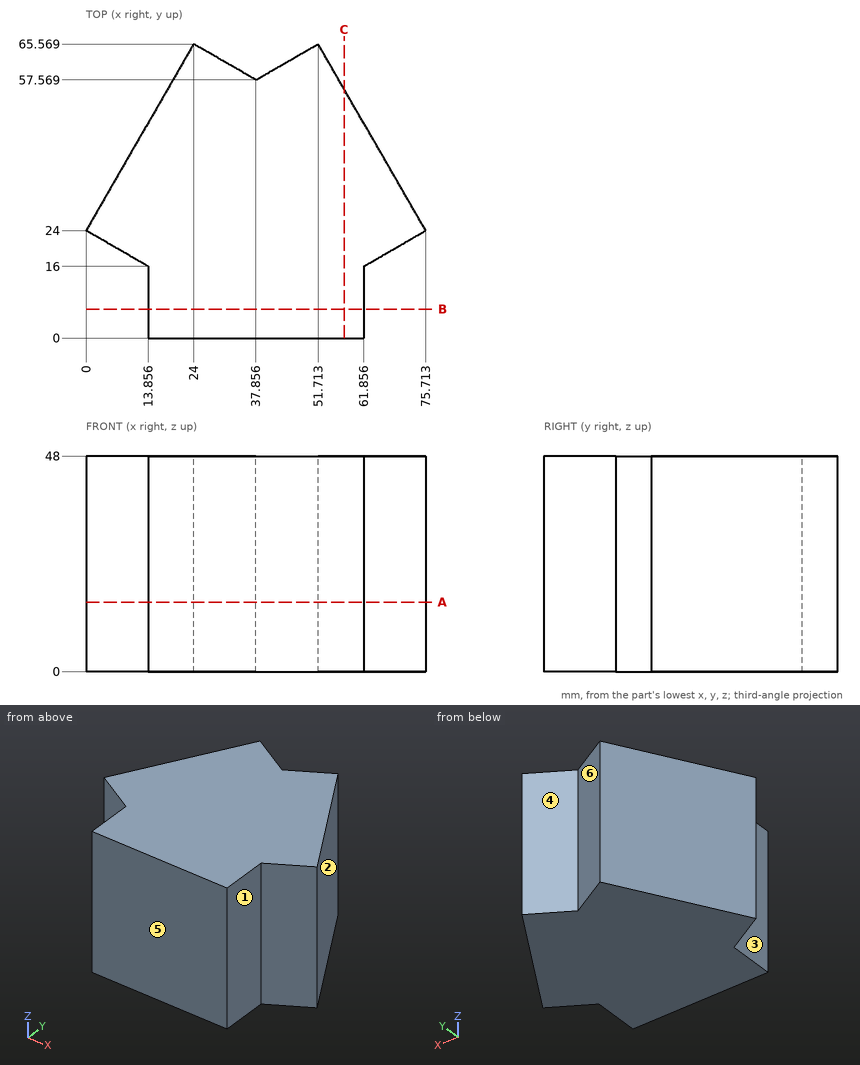
Drawing for the job (mm, zero at the part's lowest x, y, z). A direction names the side the tool comes from. Give positions to 0.01 mm unless a question says otherwise; leave off trailing zeros. Order: outer loops, then holes, each group sorted by start corner. A loop starts at its lowest first (then second) coordinate and runs counter-clockwise, first axis right, second up. Notation, with made-up numbers: M -38,-39 L -26,-39 A26 cw -26,-16 Z; hole C 73.5,58 d2. An arc over 180 degrees is marked long. Put each result on its own line as item: value. Start each with the question number.
(1) Saw through at C-C, the plane x = 57.5. Write the cut outline in (y, z) (1 decimal), then the cut area to 3 significant figures.
(2) Saw through at A-A, the plane z = 15.5. Write the cut outline in (x, y).
(3) Flat gauge pins, fed straight in: pin 1 Ø13 at (y, z) = (6.5, 15) entering from -X; pin 2 Ø8 at (y, z) = (7.5, 32.5) entering from +X; pin 3 Ø3 at (y, z) = (56, 12.5) entering from -X; pin 4 Ø3 at (x, y) = (23.5, 42.5) entering from -Z. Where does each tip first touch, or does it go through?
(4) Saw through at B-B, the plane y = 6.5. Write the cut outline in (x, z).
(5) Drill centre lines: line 1 along X through (y, z) = (8.5, 10); line 2 along X through (y, z) = (60, 10) (1 decimal); line 3 along X through (y, z) = (25, 6) (1 decimal). Where is each one in solid material? Low to high.
(6) Which spindle directions (+Z, -Z, +X, -X, +Y, -Y) get a long thin tool onto all of the face, cutting with end or side? Do the marked faces 1 and 2. Say none if no direction does.
(7) Mould opens along X. For the marked faces 3, 4, 5 and 6 say: +X half, -X half, draft (parallel to the pull), parting line (faces both ways), or undercut.
Check result:
1. outline: M 0,0 L 55.5,0 L 55.5,48 L 0,48 Z
1. area: 2,670 mm2
2. outline: M 0,24 L 13.86,16 L 13.86,0 L 61.86,0 L 61.86,16 L 75.71,24 L 51.71,65.57 L 37.86,57.57 L 24,65.57 Z
3. pin 1: stops at x = 13.86
3. pin 2: stops at x = 61.86
3. pin 3: stops at x = 17.61
3. pin 4: stops at z = 0
4. outline: M 13.86,0 L 61.86,0 L 61.86,48 L 13.86,48 Z
5. line 1: x = 13.86 to 61.86
5. line 2: x = 20.8 to 33.6, 42.1 to 54.9
5. line 3: x = 0.6 to 75.1
6. face 1: +Z, -Z, +X, -Y
6. face 2: +Z, -Z, +X, +Y
7. face 3: -X half
7. face 4: undercut
7. face 5: draft
7. face 6: undercut
